Design review of the part built by this model. Coordinates are the model's own, in mm. A direction names the side the tool comes from. Coordinates: 2 decimals unless noted, no trailing zeros. Write each loop counter-clockwise with the first axis right and the second up, starting at its lowest first coordinate (ties: lowest second). Pieces come first, ordered by that corner, then holes. Notation, with made-up numbers: M 1.25,89.25 L 43.25,89.25 A10 cw 43.25,106.25 Z; hole C 31,49 d7. An arc over 180 degrees is marked long. Write item = value, one per line.
```python
from build123d import *

# Parameters (mm, degrees)
SKETCH_1_W                   = 45
SKETCH_1_H                   = 44
EXTRUDE_1_DEPTH              = 8
CUT_EXTRUDE_1_DEPTH          = 10
FILLET_1_R                   = 3
HOLE_WIZARD_M4_1_D           = 4.5
HOLE_WIZARD_M4_1_CBORE_D     = 8
HOLE_WIZARD_M4_1_CBORE_DEPTH = 4.4
CUT_EXTRUDE_2_DEPTH          = 4
FILLET_2_R                   = 1.5
HOLE_WIZARD_13_0_13_1_D      = 13
HOLE_WIZARD_13_0_13_1_DEPTH  = 12
HOLE_WIZARD_13_0_13_1_TIP    = 3.905594024
CUT_EXTRUDE_3_DEPTH          = 5
HOLE_WIZARD_5_3_5_3_1_D      = 5.3
HOLE_WIZARD_5_3_5_3_1_DEPTH  = 12
HOLE_WIZARD_5_3_5_3_1_TIP    = 1.59228064
SKETCH_19_R                  = 4.5
CUT_EXTRUDE_4_DEPTH          = 1
HOLE_WIZARD_M3_1_D           = 2.5
HOLE_WIZARD_3_0_3_1_D        = 3
HOLE_WIZARD_3_0_3_1_DEPTH    = 40
HOLE_WIZARD_3_0_3_1_TIP      = 0.901290929
FILLET_3_R                   = 1.5


with BuildPart() as part:
    # 草图1 → 凸台-拉伸1 (new body)
    with BuildSketch(Plane.XY):
        with BuildLine():
            Line((128.173730269, 22.5), (58.173730269, 22.5))
            Line((58.173730269, 22.5), (23.173730269, 30))
            Line((23.173730269, 30), (-47.847112114, 30))
            ThreePointArc((-47.847112114, 30), (-71.826269731, 25), (-95.805427348, 30))
            Line((-95.805427348, 30), (-126.826269731, 30))
            Line((-126.826269731, 30), (-126.826269731, -30))
            Line((-126.826269731, -30), (-95.805427348, -30))
            ThreePointArc((-95.805427348, -30), (-71.826269731, -25), (-47.847112114, -30))
            Line((-47.847112114, -30), (23.173730269, -30))
            Line((23.173730269, -30), (58.173730269, -22.5))
            Line((58.173730269, -22.5), (128.173730269, -22.5))
            ThreePointArc((128.173730269, -22.5), (150.673730269, 0), (128.173730269, 22.5))
        make_face()
        with BuildLine():
            Line((-96.826269731, 12.5), (-46.826269731, 12.5))
            ThreePointArc((-46.826269731, 12.5), (-34.326269731, 0), (-46.826269731, -12.5))
            Line((-46.826269731, -12.5), (-96.826269731, -12.5))
            ThreePointArc((-96.826269731, -12.5), (-109.326269731, 0), (-96.826269731, 12.5))
        make_face(mode=Mode.SUBTRACT)
        with Locations((7.673730269, 0)):
            Rectangle(SKETCH_1_W, SKETCH_1_H, mode=Mode.SUBTRACT)
    extrude(amount=EXTRUDE_1_DEPTH)

    # 草图2 → 切除-拉伸1 (cut)
    with BuildSketch(Plane.XY.offset(8)):
        with BuildLine():
            Line((50.673730269, 10), (88.173730269, 10))
            ThreePointArc((88.173730269, 10), (98.173730269, 0), (88.173730269, -10))
            Line((88.173730269, -10), (50.673730269, -10))
            ThreePointArc((50.673730269, -10), (40.673730269, 0), (50.673730269, 10))
        make_face()
    extrude(amount=-CUT_EXTRUDE_1_DEPTH, mode=Mode.SUBTRACT)

    # 圆角1
    fillet_1_edges = [part.edges().sort_by_distance(p)[0] for p in [
        (-14.826269731, 22, 4),
        (-14.826269731, -22, 4),
        (30.173730269, -22, 4),
        (30.173730269, 22, 4),
    ]]
    fillet(fillet_1_edges, radius=FILLET_1_R)

    # M4 六角凹头螺钉的柱形沉头孔1 (through all)
    with Locations(Plane.XY.offset(8)):
        with Locations((-121.826269731, 0), (-121.826269731, -24), (-121.826269731, 24), (-95.826269731, 25), (-95.826269731, -25), (-15.826269731, -25), (-15.826269731, 25), (69.173730269, 17.5), (69.173730269, -17.5)):
            CounterBoreHole(HOLE_WIZARD_M4_1_D / 2, HOLE_WIZARD_M4_1_CBORE_D / 2, HOLE_WIZARD_M4_1_CBORE_DEPTH)

    # 草图11 → 切除-拉伸2 (cut)
    # profile 1 of 3: a face of its own
    with BuildSketch(Plane(origin=(0, 0, 0), x_dir=(-1, 0, 0), z_dir=(0, 0, -1))):
        with BuildLine():
            Line((24.826269731, -27), (47.229521978, -27))
            ThreePointArc((47.229521978, -27), (68.326801608, -22.097267763), (89.837715012, -24.629578112))
            ThreePointArc((89.837715012, -24.629578112), (96.011569063, -19.002862003), (101.826269731, -25))
            Line((101.826269731, -25), (101.826269731, -27))
            Line((101.826269731, -27), (114.826269731, -27))
            Line((114.826269731, -27), (114.826269731, 27))
            Line((114.826269731, 27), (101.826269731, 27))
            Line((101.826269731, 27), (101.826269731, 25))
            ThreePointArc((101.826269731, 25), (96.011569063, 19.002862003), (89.837715012, 24.629578112))
            ThreePointArc((89.837715012, 24.629578112), (68.326801608, 22.097267763), (47.229521978, 27))
            Line((47.229521978, 27), (24.826269731, 27))
            Line((24.826269731, 27), (24.826269731, -27))
        make_face()
        with BuildLine():
            Line((96.826269731, 15.5), (46.826269731, 15.5))
            ThreePointArc((46.826269731, 15.5), (31.326269731, 0), (46.826269731, -15.5))
            Line((46.826269731, -15.5), (96.826269731, -15.5))
            ThreePointArc((96.826269731, -15.5), (112.326269731, 0), (96.826269731, 15.5))
        make_face(mode=Mode.SUBTRACT)
    # profile 2 of 3: a face of its own
    with BuildSketch(Plane(origin=(0, 0, 0), x_dir=(-1, 0, 0), z_dir=(0, 0, -1))):
        with BuildLine():
            Line((-88.173730269, 20.25), (-115.477066498, 20.25))
            Line((-115.477066498, 20.25), (-115.477066498, 9.921609041))
            ThreePointArc((-115.477066498, 9.921609041), (-113.633917887, 6.945318766), (-112.477066498, 3.64120081))
            Line((-112.477066498, 3.64120081), (-100.65337997, 3.64120081))
            ThreePointArc((-100.65337997, 3.64120081), (-95.973229915, 10.400375246), (-88.173730269, 13))
            Line((-88.173730269, 13), (-88.173730269, 20.25))
        make_face()
    # profile 3 of 3: a face of its own
    with BuildSketch(Plane(origin=(0, 0, 0), x_dir=(-1, 0, 0), z_dir=(0, 0, -1))):
        with BuildLine():
            Line((-115.244901013, -19.5), (-88.173730269, -19.5))
            Line((-88.173730269, -19.5), (-88.173730269, -13))
            ThreePointArc((-88.173730269, -13), (-95.668248617, -10.622249984), (-100.421214485, -4.35879919))
            Line((-100.421214485, -4.35879919), (-112.244901013, -4.35879919))
            ThreePointArc((-112.244901013, -4.35879919), (-113.444814316, -7.468986993), (-115.244901013, -10.274828753))
            Line((-115.244901013, -10.274828753), (-115.244901013, -19.5))
        make_face()
    extrude(amount=-CUT_EXTRUDE_2_DEPTH, mode=Mode.SUBTRACT)

    # 圆角2
    fillet_2_edges = [part.edges().sort_by_distance(p)[0] for p in [
        (115.477066498, 9.921609041, 2),
        (115.477066498, 20.25, 2),
        (88.173730269, 20.25, 2),
        (88.173730269, 13, 2),
        (100.65337997, 3.64120081, 2),
        (112.477066498, 3.64120081, 2),
        (-24.826269731, -27, 2),
        (-24.826269731, 27, 2),
        (-47.229521978, 27, 2),
        (-89.837715012, 24.629578112, 2),
        (-101.826269731, 27, 2),
        (-114.826269731, 27, 2),
        (-114.826269731, -27, 2),
        (-101.826269731, -27, 2),
        (-89.837715012, -24.629578112, 2),
        (-47.229521978, -27, 2),
        (100.421214485, -4.35879919, 2),
        (88.173730269, -13, 2),
        (88.173730269, -19.5, 2),
        (115.244901013, -19.5, 2),
        (115.244901013, -10.274828753, 2),
        (112.244901013, -4.35879919, 2),
    ]]
    fillet(fillet_2_edges, radius=FILLET_2_R)

    # Ø13.0 (13) 直径孔1
    with Locations(Plane.XY.offset(8)):
        with Locations((128.173730269, 0)):
            Hole(HOLE_WIZARD_13_0_13_1_D / 2, depth=HOLE_WIZARD_13_0_13_1_DEPTH)
            with Locations((0, 0, -(HOLE_WIZARD_13_0_13_1_DEPTH + HOLE_WIZARD_13_0_13_1_TIP / 2))):  # 118° drill point
                Cone(0, HOLE_WIZARD_13_0_13_1_D / 2, HOLE_WIZARD_13_0_13_1_TIP, mode=Mode.SUBTRACT)

    # 草图14 → 切除-拉伸3 (cut)
    with BuildSketch(Plane(origin=(0, 0, 0), x_dir=(-1, 0, 0), z_dir=(0, 0, -1))):
        with BuildLine():
            Line((-139.173730269, 14.247806849), (-139.173730269, -14.247806849))
            ThreePointArc((-139.173730269, -14.247806849), (-128.173730269, -18), (-117.173730269, -14.247806849))
            Line((-117.173730269, -14.247806849), (-117.173730269, 14.247806849))
            ThreePointArc((-117.173730269, 14.247806849), (-128.173730269, 18), (-139.173730269, 14.247806849))
        make_face()
    extrude(amount=-CUT_EXTRUDE_3_DEPTH, mode=Mode.SUBTRACT)

    # Ø5.3 (5.3) 直径孔1
    with Locations(Plane.XY.offset(8)):
        with Locations((128.173730269, 13), (128.173730269, -13)):
            Hole(HOLE_WIZARD_5_3_5_3_1_D / 2, depth=HOLE_WIZARD_5_3_5_3_1_DEPTH)
            with Locations((0, 0, -(HOLE_WIZARD_5_3_5_3_1_DEPTH + HOLE_WIZARD_5_3_5_3_1_TIP / 2))):  # 118° drill point
                Cone(0, HOLE_WIZARD_5_3_5_3_1_D / 2, HOLE_WIZARD_5_3_5_3_1_TIP, mode=Mode.SUBTRACT)

    # 草图19 → 切除-拉伸4 (cut)
    with BuildSketch(Plane.XY.offset(8)):
        with Locations((128.173730269, 13)):
            Circle(SKETCH_19_R)
        with Locations((128.173730269, -13)):
            Circle(SKETCH_19_R)
    extrude(amount=-CUT_EXTRUDE_4_DEPTH, mode=Mode.SUBTRACT)

    # M3 螺纹孔1 (through all)
    with Locations(Plane.XY.offset(8)):
        with Locations((143.173730269, -6)):
            Hole(HOLE_WIZARD_M3_1_D / 2)

    # Ø3.0 (3) 直径孔1
    with Locations(Plane.XY.offset(8)):
        with Locations((143.173730269, 4)):
            Hole(HOLE_WIZARD_3_0_3_1_D / 2, depth=HOLE_WIZARD_3_0_3_1_DEPTH)
            with Locations((0, 0, -(HOLE_WIZARD_3_0_3_1_DEPTH + HOLE_WIZARD_3_0_3_1_TIP / 2))):  # 118° drill point
                Cone(0, HOLE_WIZARD_3_0_3_1_D / 2, HOLE_WIZARD_3_0_3_1_TIP, mode=Mode.SUBTRACT)

    # 圆角3
    fillet_3_edges = [part.edges().sort_by_distance(p)[0] for p in [
        (117.173730269, -14.247806849, 2.5),
        (139.173730269, -14.247806849, 2.5),
        (139.173730269, 14.247806849, 2.5),
        (117.173730269, 14.247806849, 2.5),
    ]]
    fillet(fillet_3_edges, radius=FILLET_3_R)


solid = part.part
```
Q1. Wall thickness on line 1 (Y direction, x = -71.5, z = 2.5); line 2 (Y direction, x = 128, z = 6.75); line 3 (X direction, y = -18, z = 7): over which ranges is each line inside the solid? List them lowest first.
Check result:
line_1 = -25 to -22, -15.5 to -12.5, 12.5 to 15.5, 22 to 25
line_2 = -22.5 to -15.64, -10.36 to -6.5, 6.5 to 10.36, 15.64 to 22.5
line_3 = -126.83 to -14.83, 30.17 to 65.21, 73.14 to 141.67
Q2. The part is to be moulded in two halves that separate along X. For faces 1 (the flat face through (40.429, -26.302, 3.944)), 2 (the flat face through (32, 0, 0)), 3 (the cylindrical face through (-96.623, -19.053, 1.972)), say which applies: +X half, -X half, draft (parallel to the pull), parting line (faces both ways), or undercut.
Check result:
face_1 = +X half
face_2 = draft
face_3 = undercut
Q3. Consider section B-B, the plane z = 2.25. State how many separate pieces and enclosed holes the cut face has, and give its area (3 significant figures).
Check result:
separate_pieces = 2
enclosed_holes = 18
area = 6,040 mm²
Q4. Consider section A-A, the plane x = 5.5. State the section outline as (y, z) points, and give its area (3 significant figures).
Check result:
outline = M -30,0 L -22,0 L -22,8 L -30,8 Z; M 22,0 L 30,0 L 30,8 L 22,8 Z
area = 128 mm²
Q5. For P1, Ø2.5, axis at x = -17, y = 25, coming from the +Z side; P2, Ø4.5, axis at y = 6, z = 2.5, coming from the +X side; P3, Ø4, axis at x = 82.5, z = 4.5, coming from the -Y side; P4, Ø3, axis at x = -11.5, y = -12, coming from the -Z side, all flat-tipped, find the tip position at first contact; note any pin that passes through.
Check result:
P1 = 3.6
P2 = 150.36
P3 = -22.5
P4 = through
Q6. Machinability: for faces 4 (the flat face through (139.174, 0, 2)), 5 (the flat face through (-13, -30, 4)), 6 (the flat face through (-14, -27, 3.6)), 7 (the flat face through (7, 22, 4)), which of the approach directions +Z, -Z, +X, -X, +Y, -Y give a long, thin tool a straight path to every point of the face, cutting with its end or side? Answer none if there is none.
Check result:
face_4 = -Z
face_5 = +Z, -Z, +X, -X, -Y
face_6 = +Z
face_7 = +Z, -Z
